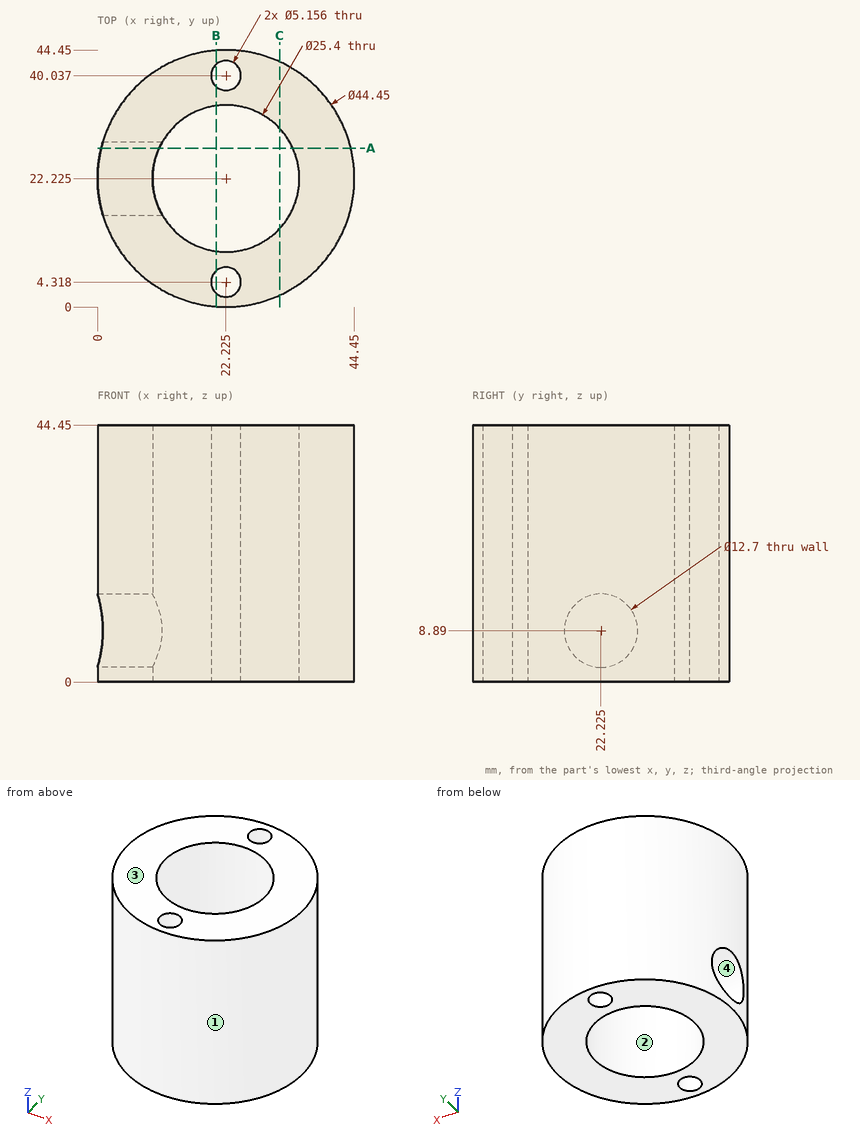
Input: dimensioned drawing with shaded views. Units: mm. Origin: part minimum x, y, z. Coordinates: 2 decimals unless noted, no trailing zeros. Order: outer loops, then holes, each group sorted by start corner. A loop starts at its lowest first (then second) coordinate and runs counter-clockwise, first axis right, second up. Notation, with made-up numbers: (-10, 77.25) -> (30, 77.25) arc R22 cw to (30, 116.25) -> close; hole circle Ø5 at (83.25, -18). An arc over 180 degrees is marked (long way). Use CSV: the item, a comma, the result in double quotes.
1) Section A-A on y = 27.5. State how many separate pieces and enclosed holes the cut face has, then the cut area to 3 significant figures.
Findings:
separate pieces,"3"
enclosed holes,"0"
area,"821 mm^2"
2) Pin query (flat end, axial travel): pin 1 Ø4 at (x, z) = (6, 22) entering from -Y; pin 2 Ø5 at (x, z) = (37, 32.5) entering from +Y; pin 3 Ø4 at (x, y) = (22.225, 4.318) entering from -Z; pin 4 Ø2 at (y, z) = (35.5, 26.5) entering from +X. Return the tip coordinate at first contact, or that it passes through.
Findings:
pin 1,"stops at y = 5.15"
pin 2,"stops at y = 40.75"
pin 3,"passes through"
pin 4,"stops at x = 40.75"
3) Section C-C on x = 31.5. Output: boundary loops of the cut face in (y, z).
Findings:
outline,"(2.03, 0) -> (13.55, 0) -> (13.55, 44.45) -> (2.03, 44.45) -> close; (30.9, 0) -> (42.42, 0) -> (42.42, 44.45) -> (30.9, 44.45) -> close"
4) Mould query, pull axis Y, two halves, no side actions, for the marked faces 1, 2, 3 and 4. Classes: +Y half, -Y half, draft (parallel to the pull), parting line (faces both ways), or undercut.
Findings:
face 1,"parting line"
face 2,"undercut"
face 3,"draft"
face 4,"undercut"
5) Line query: line 1 (Y direction, x = 24, z = 7); line 2 (Y direction, x = 23, z = 37.5) (1 decimal); line 3 (X direction, y = 38.5, z = 35) (1 decimal). Output: solid intervals per line, ascending.
Findings:
line 1,"y = 0.07 to 2.45, 6.19 to 9.65, 34.8 to 38.17, 41.91 to 44.38"
line 2,"y = 0 to 1.9, 6.8 to 9.5, 34.9 to 37.6, 42.5 to 44.4"
line 3,"x = 7.1 to 20.2, 24.3 to 37.4"
6) Section B-B on x = 20.5. Output: boundary loops of the cut face in (y, z).
Findings:
outline,"(0.07, 0) -> (2.4, 0) -> (2.4, 44.45) -> (0.07, 44.45) -> close; (6.23, 0) -> (9.64, 0) -> (9.64, 44.45) -> (6.23, 44.45) -> close; (34.81, 0) -> (38.12, 0) -> (38.12, 44.45) -> (34.81, 44.45) -> close; (41.95, 0) -> (44.38, 0) -> (44.38, 44.45) -> (41.95, 44.45) -> close"
